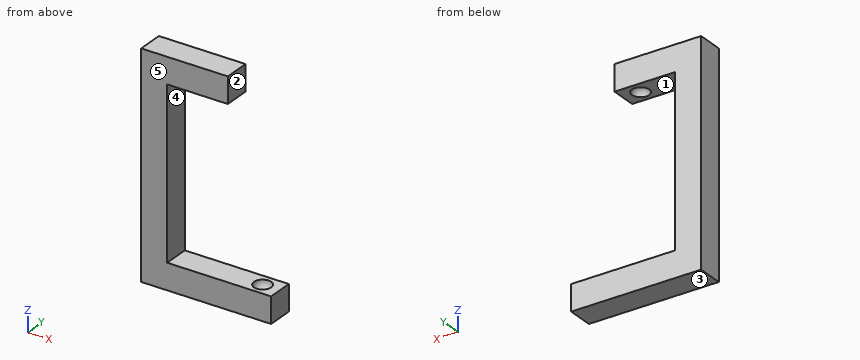
from build123d import *

# Parameters (mm, degrees)
F1_DEPTH = 15


with BuildPart() as f1:
    # F0 (on Front) → F1 (new body, symmetric)
    with BuildSketch(Plane.XZ):
        Polygon((0, 0), (0, 30), (-120, 30), (-120, 223.6491673104), (-50, 223.6491673104), (-50, 253.6491673104), (-150, 253.6491673104), (-150, 0), align=None)
    extrude(amount=F1_DEPTH, both=True)

    # F2 (on Front) → F3 (revolve, cut)
    with BuildSketch(Plane.XZ):
        with BuildLine():
            Line((-22.5, 39.6824583655), (-17.5, 20.3175416345))
            ThreePointArc((-17.5, 20.3175416345), (-10.3175416345, 32.5), (-22.5, 39.6824583655))
        make_face()
        with BuildLine():
            Line((-72.5, 233.3316256759), (-67.5, 213.9667089449))
            ThreePointArc((-67.5, 213.9667089449), (-60.3175416345, 226.1491673104), (-72.5, 233.3316256759))
        make_face()
    revolve(axis=Axis((-45, 0, 126.8245836552), (-0.25, 0, 0.9682458366)), mode=Mode.SUBTRACT)


solid = f1.part
Model file for the job. Use its own axes, mm. Face numbers are marked on the shaded views. A direction names the side the tool comes from. Give positions to 0.01 mm unless a question says otherwise; leave off trailing zeros. Order: outer loops, then holes, each group sorted by start corner. A loop starts at its lowest first (then second) coordinate and runs counter-clockwise, first axis right, second up. Notation, with made-up numbers: (-17, -12.5) - (29, -12.5) arc R21 cw to (29, 22.5) - close; hole circle Ø10 at (52.5, -12.5). An arc over 180 degrees is marked (long way). One line per item, written item: value.
Item 1: Slice it at D-D (z = 98). List the corners of the cut face in (x, y), then the cut area to 3 significant figures.
Response values:
outline: (-150, -15) - (-120, -15) - (-120, 15) - (-150, 15) - close
area: 900 mm2
Item 2: Slice it at B-B (y = -4.5). List the corners of the cut face in (x, z).
Response values:
outline: (-150, 0) - (0, 0) - (0, 30) - (-11.07, 30) arc R8.93 cw to (-28.93, 30) - (-120, 30) - (-120, 223.65) - (-78.93, 223.65) arc R8.93 cw to (-61.07, 223.65) - (-50, 223.65) - (-50, 253.65) - (-150, 253.65) - close
Item 3: Two-plate mould, pull along Z, no slides. Class the marked faces 1, 2 and 3: released by +Z, released by -Z, zero draft, split by the parting line, or undercut.
Response values:
face 1: undercut
face 2: zero draft
face 3: released by -Z
Item 4: Slice it at C-C (z = 229). List the corners of the cut face in (x, y).
Response values:
outline: (-150, -15) - (-50, -15) - (-50, 15) - (-150, 15) - close; hole circle Ø16.9 at (-70, 0)
Item 5: Tool access for the marked faces 4 and 5: list every direction of +Z, -Z, +X, -X, +Y, -Y with a clear straight run to the whole face (end or side of a thin tool).
Response values:
face 4: +X, +Y, -Y
face 5: +Z, -Z, +X, -X, -Y
Item 6: Pin check, flat tips, straight feed: pin 1 Ø2 at (y, z) = (3.5, 143) entering from +X; pin 2 Ø8 at (x, y) = (-38, 4) entering from +Z; pin 3 Ø12 at (x, y) = (-56.5, -0.5) entering from -Z. Stop position of each tip, or through.
Response values:
pin 1: x = -120
pin 2: z = 30
pin 3: z = 0
Item 7: Slice it at A-A (x = -96.5). List the corners of the cut face in (y, z).
Response values:
outline: (-15, 0) - (15, 0) - (15, 30) - (-15, 30) - close; (-15, 223.65) - (15, 223.65) - (15, 253.65) - (-15, 253.65) - close
Item 8: Wall check: line 1 (Z direction, x = -99.5, y = 9.75); line 2 (X direction, y = -9.25, z = 72); line 3 (Z direction, x = -15.5, y = 13.5). Give the ranges that are in metal, low to high.
Response values:
line 1: 0 to 30, 223.65 to 253.65
line 2: -150 to -120
line 3: 0 to 30
